```python
from build123d import *

# Parameters (mm, degrees)
SKETCH_1_W          = 88
SKETCH_1_H          = 85
EXTRUDE_1_DEPTH     = 3
SKETCH_2_R          = 1.75
SKETCH_2_R_2        = 1.1
SKETCH_2_W          = 5.1
SKETCH_2_H          = 40.2
SKETCH_2_R_3        = 2.25
SKETCH_2_W_2        = 28
SKETCH_2_H_2        = 45
CUT_EXTRUDE_1_DEPTH = 3
M2X0_4_1_D          = 1.6
M2X0_4_1_DEPTH      = 6
M2X0_4_1_TIP        = 0.480688495
CUT_EXTRUDE_2_DEPTH = 4
FILLET_7_R          = 3
FILLET_6_R          = 1.2


with BuildPart() as part:
    # ｽｹｯﾁ1 → ﾎﾞｽ - 押し出し1 (new body)
    with BuildSketch(Plane(origin=(0, 0, 0), x_dir=(1, 0, 0), z_dir=(0, 1, 0))):
        Rectangle(SKETCH_1_W, SKETCH_1_H)
    extrude(amount=EXTRUDE_1_DEPTH)

    # ｽｹｯﾁ2 → ｶｯﾄ - 押し出し1 (cut)
    with BuildSketch(Plane(origin=(0, 3, 0), x_dir=(1, 0, 0), z_dir=(0, 1, 0))):
        with Locations((-26.5, 27.5)):
            Circle(SKETCH_2_R)
        with Locations((26.5, 27.5)):
            Circle(SKETCH_2_R)
        with Locations((-28.45, -24.5)):
            Circle(SKETCH_2_R_2)
        with Locations((-24.55, -24.5)):
            Circle(SKETCH_2_R_2)
        with Locations((-26.5, -5)):
            Rectangle(SKETCH_2_W, SKETCH_2_H)
        with Locations((-28.45, 14.5)):
            Circle(SKETCH_2_R_2)
        with Locations((-24.55, 14.5)):
            Circle(SKETCH_2_R_2)
        with Locations((26.5, -5)):
            Rectangle(SKETCH_2_W, SKETCH_2_H)
        with Locations((24.55, 14.5)):
            Circle(SKETCH_2_R_2)
        with Locations((28.45, 14.5)):
            Circle(SKETCH_2_R_2)
        with Locations((24.55, -24.5)):
            Circle(SKETCH_2_R_2)
        with Locations((28.45, -24.5)):
            Circle(SKETCH_2_R_2)
        with Locations((-26.5, -37.5)):
            Circle(SKETCH_2_R)
        with Locations((26.5, -37.5)):
            Circle(SKETCH_2_R)
        with Locations((-36.5, -25)):
            Circle(SKETCH_2_R_3)
        with Locations((-36.5, 35)):
            Circle(SKETCH_2_R_3)
        with Locations((36.5, 35)):
            Circle(SKETCH_2_R_3)
        with Locations((36.5, -25)):
            Circle(SKETCH_2_R_3)
        with Locations((0, -5)):
            Rectangle(SKETCH_2_W_2, SKETCH_2_H_2)
    extrude(amount=-CUT_EXTRUDE_1_DEPTH, mode=Mode.SUBTRACT)

    # M2x0.4 ねじ穴1
    with Locations(Plane(origin=(0, 3, 0), x_dir=(1, 0, 0), z_dir=(0, 1, 0))):
        with Locations((-10, 32.5), (10, 32.5)):
            Hole(M2X0_4_1_D / 2, depth=M2X0_4_1_DEPTH)
            with Locations((0, 0, -(M2X0_4_1_DEPTH + M2X0_4_1_TIP / 2))):  # 118° drill point
                Cone(0, M2X0_4_1_D / 2, M2X0_4_1_TIP, mode=Mode.SUBTRACT)

    # ｽｹｯﾁ5 → ｶｯﾄ - 押し出し2 (cut, through all)
    with BuildSketch(Plane(origin=(0, 3, 0), x_dir=(1, 0, 0), z_dir=(0, 1, 0))):
        Polygon((-5.5, 42.5), (5.5, 42.5), (5.5, 26.5), (8, 26.5), (8, 22.5), (-8, 22.5), (-8, 26.5), (-5.5, 26.5), align=None)
    extrude(amount=-CUT_EXTRUDE_2_DEPTH, mode=Mode.SUBTRACT)

    # ﾌｨﾚｯﾄ7
    fillet_7_edges = [part.edges().sort_by_distance(p)[0] for p in [
        (-5.5, 1.5, -42.5),
        (5.5, 1.5, -42.5),
        (-14, 1.5, -17.5),
        (14, 1.5, -17.5),
        (14, 1.5, 27.5),
        (-14, 1.5, 27.5),
        (44, 1.5, 42.5),
        (-44, 1.5, 42.5),
    ]]
    fillet(fillet_7_edges, radius=FILLET_7_R)

    # ﾌｨﾚｯﾄ6
    fillet_6_edges = [part.edges().sort_by_distance(p)[0] for p in [
        (5.5, 1.5, -26.5),
        (8, 1.5, -26.5),
        (8, 1.5, -22.5),
        (-8, 1.5, -22.5),
        (-8, 1.5, -26.5),
        (-5.5, 1.5, -26.5),
    ]]
    fillet(fillet_6_edges, radius=FILLET_6_R)


solid = part.part
```
Source: CAD feature listing. Evaluate the final solid. Frame: model axes, mm. A direction names the side the tool comes from. Give positions to 0.01 mm unless a question says otherwise; leave off trailing zeros. Write each loop counter-clockwise with the first axis right and the second up, starting at its lowest first coordinate (ties: lowest second). Pieces come first, ordered by that corner, then holes.
1. Access query for faces 1 (the face through (-20, 3, -1)), 2 (the face through (29.05, 2, 5)), 3 (the face through (-6.4, 1.48, -41.64)). Directions: +Z, -Z, +X, -X, +Y, -Y. A direction counts if a zero-diameter tool reaches every point of the face in a straight line with its end or side. Return the directions, or none.
2. Section query D-D (y = 1.4). Count the separate pieces of the cut face and the enclosed holes in it, then the cut area to 3 significant figures.
3. Material intervals for line 1 along Z through (x, y) = (-26.5, 1.25); line 2 along X through (y, z) = (2.7, -6); line 3 along Z through (x, y) = (-10, 2.6), sorted ascending.
4. First-contact query: pin 1 (1.5 mm diameter, centred on x = 5.5, y = 2.5, fed in from -Z). Flat tip, straight axial feed; report the tip coordinate or a pass-through.
5. Section query C-C (x = 26.5). Return the cut outline in (y, z).
6. Section query B-B (x = -1). Return the cut outline in (y, z), then the cut area to 3 significant figures.
7. Section query A-A (z = -35). Return the cut outline in (x, y).
8. Pull-direction query (X, two-part tool) for faces 4 (the face through (25.21, 1.52, -28.68)), 5 (the face through (-26, 1, -42.5)); classes: +X half, -X half, draft (parallel to the pull), parting line (faces both ways), or undercut.
Output values:
1. face 1: +Z, -Z, +X, -X, +Y
1. face 2: +Y, -Y
1. face 3: -Z, +Y, -Y
2. separate pieces: 1
2. enclosed holes: 13
2. area: 5,450 mm2
3. line 1: z = -42.5 to -29.25, -25.75 to -15.1, 25.1 to 35.75, 39.25 to 42.5
3. line 2: x = -44 to -29.05, -23.95 to -14, 14 to 23.95, 29.05 to 44
3. line 3: z = -42.5 to -33.3, -31.7 to -17.5, 27.5 to 42.5
4. pin 1: stops at z = -41.48
5. outline: (0, -42.5) - (3, -42.5) - (3, -29.25) - (0, -29.25) - close; (0, -25.75) - (3, -25.75) - (3, -15.1) - (0, -15.1) - close; (0, 25.1) - (3, 25.1) - (3, 35.75) - (0, 35.75) - close; (0, 39.25) - (3, 39.25) - (3, 42.5) - (0, 42.5) - close
6. outline: (0, -22.5) - (3, -22.5) - (3, -17.5) - (0, -17.5) - close; (0, 27.5) - (3, 27.5) - (3, 42.5) - (0, 42.5) - close
6. area: 60.0 mm2
7. outline: (-44, 0) - (-38.75, 0) - (-38.75, 3) - (-44, 3) - close; (-34.25, 0) - (-5.5, 0) - (-5.5, 3) - (-34.25, 3) - close; (5.5, 0) - (34.25, 0) - (34.25, 3) - (5.5, 3) - close; (38.75, 0) - (44, 0) - (44, 3) - (38.75, 3) - close
8. face 4: undercut
8. face 5: draft
